```python
from build123d import *

# Parameters (mm, degrees)
ESQUISSE1_R                                    = 21.5
ESQUISSE1_R_2                                  = 5
ESQUISSE1_R_3                                  = 1
ESQUISSE1_R_4                                  = 1.25
BOSS_EXTRU_1_DEPTH                             = 4
FRAISAGE_POUR_VIS_T_TE_FRAIS_E_M31_D           = 3.4
FRAISAGE_POUR_VIS_T_TE_FRAIS_E_M31_CSINK_D     = 6.3
FRAISAGE_POUR_VIS_T_TE_FRAIS_E_M31_CSINK_ANGLE = 90


with BuildPart() as part:
    # Esquisse1 → Boss.-Extru.1 (new body)
    with BuildSketch(Plane(origin=(0, 0, 0), x_dir=(1, 0, 0), z_dir=(0, 1, 0))):
        with Locations(Location((0, 0, 0), (0, 0, 270))):
            Circle(ESQUISSE1_R)
        with Locations(Location((0, 0, 0), (0, 0, 270))):
            Circle(ESQUISSE1_R_2, mode=Mode.SUBTRACT)
        with Locations(Location((-5.123344298, 8.587860223, 0), (0, 0, 270))):
            Circle(ESQUISSE1_R_3, mode=Mode.SUBTRACT)
        with Locations(Location((8.587860223, 5.123344298, 0), (0, 0, 270))):
            Circle(ESQUISSE1_R_3, mode=Mode.SUBTRACT)
        with Locations(Location((5.123344298, -8.587860223, 0), (0, 0, 270))):
            Circle(ESQUISSE1_R_3, mode=Mode.SUBTRACT)
        with Locations(Location((-8.587860223, -5.123344298, 0), (0, 0, 270))):
            Circle(ESQUISSE1_R_3, mode=Mode.SUBTRACT)
        with Locations(Location((0, 19, 0), (0, 0, 270))):
            Circle(ESQUISSE1_R_4, mode=Mode.SUBTRACT)
        with Locations(Location((19, 0, 0), (0, 0, 270))):
            Circle(ESQUISSE1_R_4, mode=Mode.SUBTRACT)
        with Locations(Location((0, -19, 0), (0, 0, 270))):
            Circle(ESQUISSE1_R_4, mode=Mode.SUBTRACT)
        with Locations(Location((-19, 0, 0), (0, 0, 270))):
            Circle(ESQUISSE1_R_4, mode=Mode.SUBTRACT)
    extrude(amount=BOSS_EXTRU_1_DEPTH)

    # Fraisage pour vis à tête fraisée M31 (through all)
    with Locations(Plane(origin=(0, 4, 0), x_dir=(1, 0, 0), z_dir=(0, 1, 0))):
        with Locations((-5.123344298, 8.587860223), (8.587860223, 5.123344298), (5.123344298, -8.587860223), (-8.587860223, -5.123344298)):
            CounterSinkHole(FRAISAGE_POUR_VIS_T_TE_FRAIS_E_M31_D / 2, FRAISAGE_POUR_VIS_T_TE_FRAIS_E_M31_CSINK_D / 2, counter_sink_angle=FRAISAGE_POUR_VIS_T_TE_FRAIS_E_M31_CSINK_ANGLE)


solid = part.part
```
Can you work these out from the model? Positions are in its coordinate system, mm. Coordinates: 2 decimals unless noted, no trailing zeros. Loops run counter-clockwise (first coordinate to the right, second up) from the corner with the lowest first, then second, coordinate; pieces in that order, holes last. Notation, with made-up numbers: (75, 29) -> (118, 29) arc R13 ccw to (118, 48) -> close; hole circle Ø3 at (71, -36.75). An arc over 180 degrees is marked (long way). Put each result on its own line as item: value. Start each with the question number.
Q1. I'm going to push flat-ended pins straight in: P1, Ø2, axis at x = 0, z = -19, coming from the +Y side; P2, Ø2, axis at x = 16.5, y = 0.5, coming from the -Z side; P3, Ø5.5, axis at x = -8.59, z = 5.12, coming from the +Y side; P4, Ø1.5, axis at x = 4.5, y = 1.5, coming from the +Z side. Where does each tip first touch, or does it pass through?
Q2. I want a section at A-A (z = 0). Write out the boundary of the cut face in (x, y), plus the area to 3 significant figures.
Q3. I want a section at C-C (z = -19). Write out the boundary of the cut face in (x, y), plus the area to 3 significant figures.
Q4. If I drill on line 1 (X direction, y = 0.8, z = 0); line 2 (Z direction, x = -18.5, y = 0.6); line 3 (Z direction, x = 4, y = 3.15), over which ranges is the centre line in solid material (lowest first)? Write a range as [from, to].
Q5. I want a section at D-D (y = 3.25). Count the separate pieces of the cut face and the enclosed holes in it, plus the area to 3 significant figures.
Q6. Thinking about a two-plate mould opening in Z: for faces 1 (the face through (-4.88, 1.97, -1.08)), 2 (the face through (14.531, 1.972, -15.846)), 3 (the face through (-4, 4, 4)), which applies, pulls with the +Z half, pulls with the -Z half, needs draft (parallel to the pull), parting line crosses it, or undercut?
Q7. I want a section at B-B (x = 0). Write out the boundary of the cut face in (y, z).
Taken from the geometry:
1. P1: passes through
1. P2: stops at z = -14.9
1. P3: stops at y = 3.6
1. P4: stops at z = 21.17
2. outline: (-21.5, 0) -> (-20.25, 0) -> (-20.25, 4) -> (-21.5, 4) -> close; (-17.75, 0) -> (-5, 0) -> (-5, 4) -> (-17.75, 4) -> close; (5, 0) -> (17.75, 0) -> (17.75, 4) -> (5, 4) -> close; (20.25, 0) -> (21.5, 0) -> (21.5, 4) -> (20.25, 4) -> close
2. area: 112 mm2
3. outline: (-10.06, 0) -> (-1.25, 0) -> (-1.25, 4) -> (-10.06, 4) -> close; (1.25, 0) -> (10.06, 0) -> (10.06, 4) -> (1.25, 4) -> close
3. area: 70.5 mm2
4. line 1: x = [-21.5, -20.25], [-17.75, -5], [5, 17.75], [20.25, 21.5]
4. line 2: z = [-10.95, -1.15], [1.15, 10.95]
4. line 3: z = [-21.12, -3], [3, 6.58], [10.59, 21.12]
5. separate pieces: 1
5. enclosed holes: 9
5. area: 1,280 mm2
6. face 1: undercut
6. face 2: parting line crosses it
6. face 3: needs draft
7. outline: (0, -21.5) -> (4, -21.5) -> (4, -20.25) -> (0, -20.25) -> close; (0, -17.75) -> (4, -17.75) -> (4, -5) -> (0, -5) -> close; (0, 5) -> (4, 5) -> (4, 17.75) -> (0, 17.75) -> close; (0, 20.25) -> (4, 20.25) -> (4, 21.5) -> (0, 21.5) -> close
